The model under review builds one solid part; all positions refer to its coordinate system, in mm. Face numbers are marked on the shaded views. A direction names the side the tool comes from. Give positions to 0.01 mm unless a question says otherwise; leave off trailing zeros. Loops run counter-clockwise (first coordinate to the right, second up) from the corner with the lowest first, then second, coordinate; pieces in that order, holes last. Notation, with made-up numbers: M -19.5,14.5 L -15.5,14.5 A16 cw -15.5,42.5 Z; hole C 1.5,22.25 d1. An arc over 180 degrees is marked long. Write item = value, one per line. Start each with the question number.
1. We need section B-B on x = -49. Give the boundary of the cut face in (y, z), then the cut area to 3 significant figures.
2. For pin 1 (4 mm diameter, centred on y = 32.5, z = 32, fed in from -X); pin 2 (10 mm diameter, centred on y = 27.5, z = 64.5, fed in from +X); pin 3 (8 mm diameter, centred on x = -45, z = 32, fed in from +Y), all flat-tipped, find the tip position at first contact; note any pin that passes through.
3. Wall thickness on line 1 along Z through (x, y) = (-53.5, 26); line 2 along Y through (x, z) = (-32.5, 27.5); line 3 along X through (y, z) = (21.5, 67): over which ranges is each line inside the solid? List them lowest first. Write a range as from..to.
4. For the marked faces 1 and 2, list the 3-axis set-ups (+Z, -Z, +X, -X, +Y, -Y) from which the entire face can be reached by the end or side of a thin tool; tool diameter is ignored.
5. We need section C-C on z = 92. Give the boundary of the cut face in (x, y), then the cut area to 3 significant figures.
6. We need section A-A on y = 9. Give the boundary of the cut face in (x, z).
7. We need section D-D on y = 45.5. Give the boundary of the cut face in (x, z).
from build123d import *

# Parameters (mm, degrees)
F0_R      = 26.44498
F1_DEPTH  = 5.181627
F1_FACE_R = 26.44498
F2_DEPTH  = 55.07613
F3_R      = 17.120635
F4_DEPTH  = 110.949099


with BuildPart() as f1:
    # F0 (on Top) → F1 (new body)
    with BuildSketch(Plane.XY):
        with Locations((-31.49575, 22.197023)):
            Circle(F0_R)
    extrude(amount=F1_DEPTH)

    # F1_face (on face) → F2 (join)
    with BuildSketch(Plane(origin=(-31.49575, 22.197023, 5.181627), x_dir=(1, 0, 0), z_dir=(0, 0, 1))):
        Circle(F1_FACE_R)
    extrude(amount=F2_DEPTH)

    # F3 (on Top) → F4 (join)
    with BuildSketch(Plane.XY):
        with Locations((-33.796612, 22.234606)):
            Circle(F3_R)
    extrude(amount=F4_DEPTH)


solid = f1.part
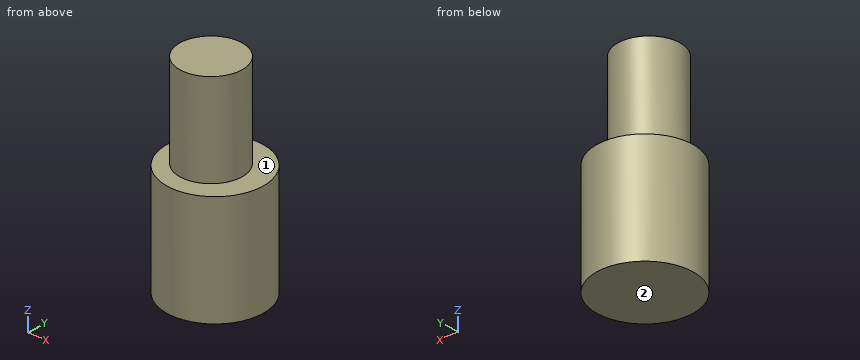
Final values:
q1.outline = M 2.37,0 L 42.02,0 L 42.02,60.26 L 30.11,60.26 L 30.11,110.95 L 14.36,110.95 L 14.36,60.26 L 2.37,60.26 Z
q1.area = 3,190 mm²
q2.pin_1 = -56.6
q2.pin_2 = -5.18
q2.pin_3 = 46.88
q3.line_1 = 0..60.26
q3.line_2 = -4.23..48.62
q3.line_3 = -50.9..-16.69
q4.face_1 = +Z
q4.face_2 = -Z, +X, -X, +Y, -Y
q5.outline = C -33.8,22.23 d34.24
q5.area = 921 mm²
q6.outline = M -54.41,0 L -8.58,0 L -8.58,60.26 L -22.94,60.26 L -22.94,110.95 L -44.66,110.95 L -44.66,60.26 L -54.41,60.26 Z
q7.outline = M -44,0 L -18.99,0 L -18.99,60.26 L -44,60.26 Z
